from build123d import *

# Parameters (mm, degrees)
F1_DEPTH = 134.62
F2_W     = 19.05
F2_H     = 8.255
F3_DEPTH = 228.6


with BuildPart() as f1:
    # F0 (on Front) → F1 (new body)
    with BuildSketch(Plane.XZ):
        Polygon((-114.3, -25.4), (114.3, -25.4), (114.3, -9.525), (66.294, 25.4), (36.197161, 25.4), (36.197161, 12.7), (-8.255, 12.7), (-8.255, 25.4), (-11.43, 25.4), (-11.43, 19.05), (-31.75, 19.05), (-31.75, 25.4), (-82.55, 25.4), (-114.3, -6.35), align=None)
    extrude(amount=F1_DEPTH)

    # F2 (on face) → F3 (cut)
    with BuildSketch(Plane.YZ.offset(114.3)):
        with Locations((-125.095, -21.2725)):
            Rectangle(F2_W, F2_H)
    extrude(amount=-F3_DEPTH, mode=Mode.SUBTRACT)


solid = f1.part
Can you work these out from the model? Positions are in its coordinate system, mm. A direction names the side the tool comes from. Coordinates: 2 decimals unless noted, no trailing zeros. Write each loop counter-clockwise with the first axis right and the second up, starting at its lowest first coordinate (ties: lowest second). Pieces come first, ordered by that corner, then holes. Notation, with made-up numbers: M 75.5,72 L 99.5,72 A9 cw 99.5,88 Z; hole C 17.5,9 d11. An arc over 180 degrees is marked long. Use one line per item in the form item = value.
Q1. If we section it at A-A (y = -118): Write out the boundary of the cut face in (x, z) (3 decimals).
Model answer:
outline = M -114.3,-17.145 L 114.3,-17.145 L 114.3,-9.525 L 66.294,25.4 L 36.197,25.4 L 36.197,12.7 L -8.255,12.7 L -8.255,25.4 L -11.43,25.4 L -11.43,19.05 L -31.75,19.05 L -31.75,25.4 L -82.55,25.4 L -114.3,-6.35 Z
Q2. For P1, Ø6.5, axis at x = 30.5, z = -20.5, coming from the -Y side; P2, Ø12, axis at x = -22, y = -107, coming from the +Z side; P3, Ø1.5, axis at y = -23.5, z = -3.5, coming from the -X side, each with a flat end and sliding along its axis, tell me the tip position at first contact or that it passes through.
Model answer:
P1 = -115.57
P2 = 19.05
P3 = -112.2
Q3. I need wall thicknesses on line 1 along X through (y, z) = (-92.5, 22) (3 decimals); line 2 along Y through (x, z) = (103, -19.5); line 3 along X through (y, z) = (-119, 23.5) (3 decimals). Which ranges of each line are inside material? Lowest first, please. Write a range as from..to.
Model answer:
line_1 = -85.95..-31.75, -11.43..-8.255, 36.197..70.967
line_2 = -115.57..0
line_3 = -84.45..-31.75, -11.43..-8.255, 36.197..68.906
Q4. If we section it at B-B (x = -98): Write out the boundary of the cut face in (y, z) (3 decimals).
Model answer:
outline = M -134.62,-17.145 L -115.57,-17.145 L -115.57,-25.4 L 0,-25.4 L 0,9.95 L -134.62,9.95 Z
Q5. For faces 1 (the flat face through (2, -125, -17.145)), 2 (the flat face through (-98.2, -66.37, 9.75)), 3 (the flat face through (36.197, -66, 19)), which set-ups out of +Z, -Z, +X, -X, +Y, -Y let a thin tool reach every point of the face, with its end or its side?
Model answer:
face_1 = -Z, +X, -X, -Y
face_2 = +Z, -X, +Y, -Y
face_3 = +Z, +Y, -Y
Q6. If we section it at C-C (z = 3.5): Write out the boundary of the cut face in (x, y), then the cut area to 3 significant figures.
Model answer:
outline = M -104.45,-134.62 L 96.4,-134.62 L 96.4,0 L -104.45,0 Z
area = 27,000 mm^2
Q7. If we section it at D-D (y = -14): Write out the boundary of the cut face in (x, z) (3 decimals).
Model answer:
outline = M -114.3,-25.4 L 114.3,-25.4 L 114.3,-9.525 L 66.294,25.4 L 36.197,25.4 L 36.197,12.7 L -8.255,12.7 L -8.255,25.4 L -11.43,25.4 L -11.43,19.05 L -31.75,19.05 L -31.75,25.4 L -82.55,25.4 L -114.3,-6.35 Z
